Here's the drawing with two shaded views (mm, measured from the low corner). I have some questions. Give positions to 0.01 mm unless a question says otherwise; leave off trailing zeros. Write each loop counter-clockwise with the first axis right and the second up, starting at its lowest first coordinate (ties: lowest second). Pieces come first, ordered by that corner, then holes.
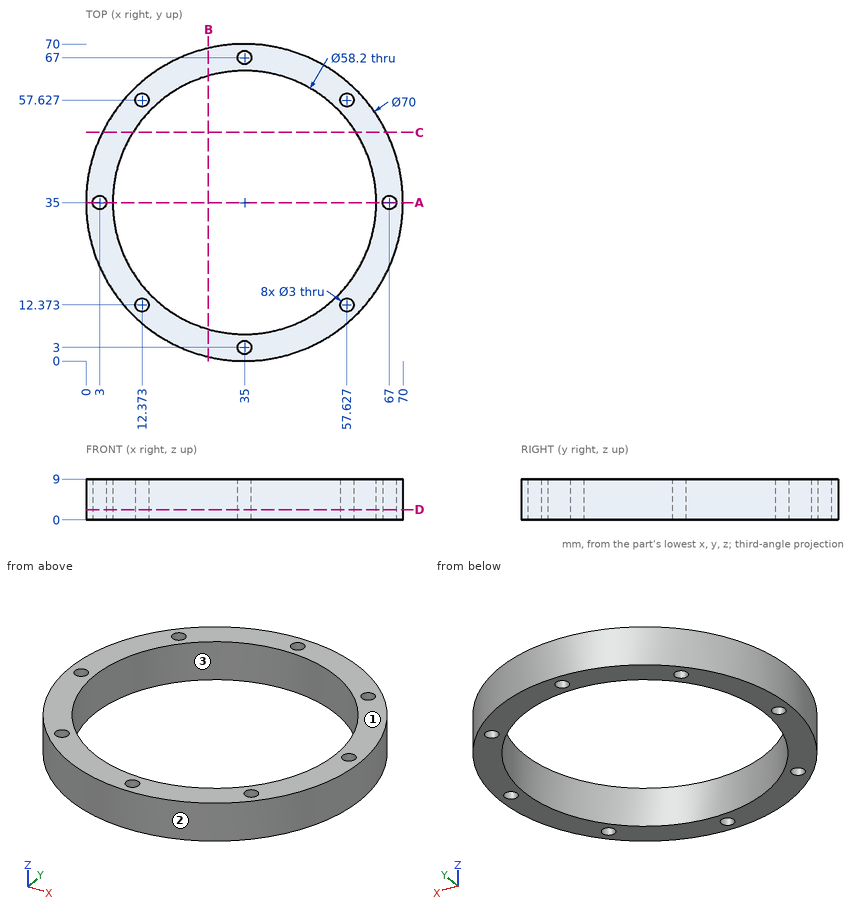
(1) If we mould it in two halves opening along Y, with no side actions, what happens to the marked faces 1, 2 and 3? For each: +Y half, -Y half, draft (parallel to the pull), parting line (faces both ways), or undercut.
Returned:
face 1: draft
face 2: parting line
face 3: undercut
(2) If I drill on L1, parallel to Y at x = 35, z = 3; L2, parallel to X at y = 58, z = 8 (1 decimal), over which ranges is the centre line in solid material (lowest first)?
Returned:
L1: y = 0 to 1.5, 4.5 to 5.9, 64.1 to 65.5, 68.5 to 70
L2: x = 8.6 to 10.9, 13.8 to 17.2, 52.8 to 56.2, 59.1 to 61.4
(3) Imagine slicing it at A-A, the plane y = 35. Write out the boundary of the cut face in (x, z).
Returned:
outline: (0, 0) - (1.5, 0) - (1.5, 9) - (0, 9) - close; (4.5, 0) - (5.9, 0) - (5.9, 9) - (4.5, 9) - close; (64.1, 0) - (65.5, 0) - (65.5, 9) - (64.1, 9) - close; (68.5, 0) - (70, 0) - (70, 9) - (68.5, 9) - close
(4) Imagine slicing it at C-C, the plane y = 50.5. Write out the boundary of the cut face in (x, z).
Returned:
outline: (3.62, 0) - (10.37, 0) - (10.37, 9) - (3.62, 9) - close; (59.63, 0) - (66.38, 0) - (66.38, 9) - (59.63, 9) - close
(5) Will these pins go through, and if not, where does the flat tip stop? P1, Ø2.5, axis at x = 57.63, y = 57.63, coming from the +Z side; P2, Ø2, axis at x = 23.5, z = 5.5, coming from the -Y side; P3, Ø5, axis at x = 13, z = 8, coming from the +Y side (1 decimal); P4, Ø5, axis at x = 23.5, z = 4, coming from the +Y side.
Returned:
P1: passes through
P2: stops at y = 1.61
P3: stops at y = 64.1
P4: stops at y = 68.82
(6) Imagine slicing it at B-B, the plane x = 27. Write out the boundary of the cut face in (y, z), plus the area to 3 significant figures.
Returned:
outline: (0.93, 0) - (7.02, 0) - (7.02, 9) - (0.93, 9) - close; (62.98, 0) - (69.07, 0) - (69.07, 9) - (62.98, 9) - close
area: 110 mm2
(7) Imagine slicing it at D-D, the plane z = 2.25. Give the number of separate pieces and of enclosed holes in the cut face, plus the area to 3 significant figures.
Returned:
separate pieces: 1
enclosed holes: 9
area: 1,130 mm2
